Work out the finished part from the listing and answer in its coordinate system (mm). Face numbers are marked on the shaded views. A direction names the side the tool comes from. Coordinates: 2 decimals unless noted, no trailing zeros. Order: outer loops, then holes, each group sorted by start corner. A loop starts at its lowest first (then second) coordinate and runs counter-clockwise, first axis right, second up.
```python
from build123d import *

# Parameters (mm, degrees)
BOSS_EXTRUDE1_DEPTH = 4.7498
SKETCH2_R           = 2.54
CUT_EXTRUDE1_DEPTH  = 4.7498
SKETCH3_W           = 38.1
SKETCH3_H           = 4.866954954
BOSS_EXTRUDE2_DEPTH = 14.3002
SKETCH4_R           = 7.1374
BOSS_EXTRUDE3_DEPTH = 38.1
SKETCH5_R           = 3.81
CUT_EXTRUDE2_DEPTH  = 43.2562


with BuildPart() as part:
    # Sketch1 → Boss-Extrude1 (new body)
    with BuildSketch(Plane(origin=(0, 0, 0), x_dir=(1, 0, 0), z_dir=(0, 1, 0))):
        Polygon((0, 0), (38.1, 0), (30.471493689, 46.0502), (7.255893689, 46.0502), align=None)
    extrude(amount=BOSS_EXTRUDE1_DEPTH)

    # Sketch2 → Cut-Extrude1 (cut)
    with BuildSketch(Plane(origin=(0, 4.7498, 0), x_dir=(1, 0, 0), z_dir=(0, 1, 0))):
        with Locations(Location((18.863693689, 36.9316, 0), (0, 0, 270))):
            Circle(SKETCH2_R)
        with Locations(Location((8.509, 10.3124, 0), (0, 0, 270))):
            Circle(SKETCH2_R)
        with Locations(Location((29.591, 10.3124, 0), (0, 0, 270))):
            Circle(SKETCH2_R)
    extrude(amount=-CUT_EXTRUDE1_DEPTH, mode=Mode.SUBTRACT)

    # Sketch3 → Boss-Extrude2 (add)
    with BuildSketch(Plane.XY):
        with Locations((19.05, 2.316322523)):
            Rectangle(SKETCH3_W, SKETCH3_H)
    extrude(amount=BOSS_EXTRUDE2_DEPTH)

    # Sketch4 → Boss-Extrude3 (add)
    with BuildSketch(Plane(origin=(38.1, 0, 0), x_dir=(0, 0, -1), z_dir=(1, 0, 0))):
        with Locations((-7.1501, 7.248845046)):
            Circle(SKETCH4_R)
    extrude(amount=-BOSS_EXTRUDE3_DEPTH)

    # Sketch5 → Cut-Extrude2 (cut)
    with BuildSketch(Plane(origin=(38.1, 0, 0), x_dir=(0, 0, -1), z_dir=(1, 0, 0))):
        with Locations((-7.1501, 8.036245046)):
            Circle(SKETCH5_R)
    extrude(amount=-CUT_EXTRUDE2_DEPTH, mode=Mode.SUBTRACT)


solid = part.part
```
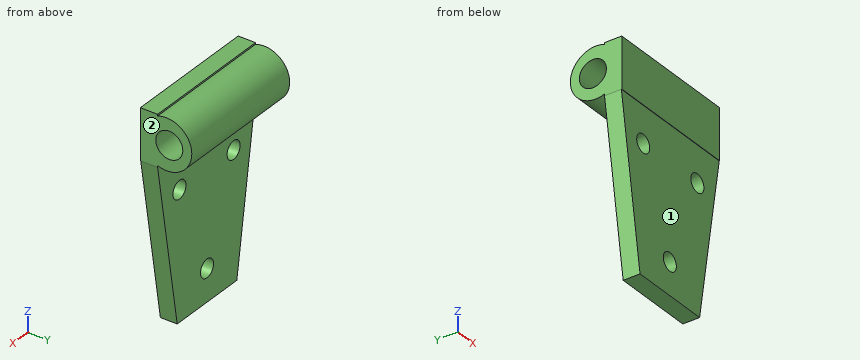
1. For the marked faces 1 and 2, determine the directions among +Z, -Z, +X, -X, +Y, -Y from which every point of the face is accessible in a straight line to the end or side of a thin tool.
2. The part is cut by section B-B (z = -38.5). Determine the outline of the cut face in (x, y).
3. Consider probe 1 along Y at (x, z) = (14.5, -9); probe 2 along Y at (x, z) = (19, 5.5); probe 3 along Y at (x, z) = (11, 10). Determine where each line is inside the solid, lowest interval first.
4. Flat-ended cylindrical pins translate along their axes: pin 1 (10 mm diameter, centred on x = 28.5, z = -9, fed in from +Y); pin 2 (8 mm diameter, centred on x = 8.51, z = -10.31, fed in from -Y); pin 3 (3 mm diameter, centred on y = 6, z = -8.5, fed in from -X); pin 4 (6 mm diameter, centred on y = 8.04, z = 7.15, fed in from +X). Find the tip coordinate at first contact, or state that the pin passes through.
5. The part is cut by section D-D (y = 3.5). Determine the outline of the cut face in (x, z).
6. The part is cut by section C-C (y = 7.25). Determine the outline of the cut face in (x, z), plus the area to 3 significant figures.
7. The part is cut by section A-A (x = 31.5). Determine the outline of the cut face in (y, z).
Worked out:
1. face 1: -Z, +X, -X, -Y
1. face 2: +Z, -Z, +X, +Y, -Y
2. outline: (6.07, 0) - (16.87, 0) - (16.87, 4.75) - (6.07, 4.75) - close; (20.86, 0) - (31.72, 0) - (31.72, 4.75) - (20.86, 4.75) - close
3. probe 1: y = 0 to 4.75
3. probe 2: y = -0.12 to 4.6, 11.47 to 14.19
3. probe 3: y = -0.12 to 5.51, 10.56 to 13.79
4. pin 1: stops at y = 4.75
4. pin 2: stops at y = 0
4. pin 3: stops at x = 1.21
4. pin 4: passes through
5. outline: (0, 0) - (7.26, -46.05) - (30.47, -46.05) - (38.1, 0) - (38.1, 14.3) - (0, 14.3) - close; hole circle Ø5.08 at (8.51, -10.31); hole circle Ø5.08 at (18.86, -36.93); hole circle Ø5.08 at (29.59, -10.31)
6. outline: (0, 0.01) - (38.1, 0.01) - (38.1, 3.42) - (0, 3.42) - close; (0, 10.88) - (38.1, 10.88) - (38.1, 14.29) - (0, 14.29) - close
6. area: 260 mm2
7. outline: (-0.12, 0) - (0, 0) - (0, -8.64) - (4.75, -8.64) - (4.75, 0.46) arc R7.14 ccw (long way) to (4.75, 13.84) - (4.75, 14.3) - (-0.12, 14.3) - close; (0, -39.84) - (4.75, -39.84) - (4.75, -11.99) - (0, -11.99) - close; hole circle Ø7.62 at (8.04, 7.15)
